Design review of the part built by this model. Coordinates are the model's own, in mm. Face numbers are marked on the shaded views. Give positions to 0.01 mm unless a question says otherwise; leave off trailing zeros.
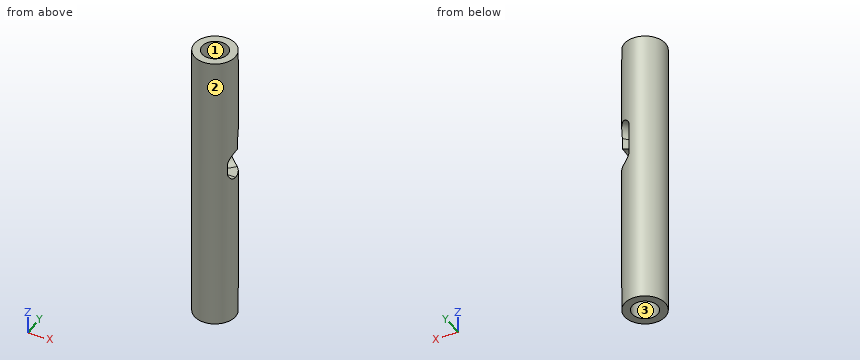
from build123d import *

# Parameters (mm, degrees)
SKETCH1_R           = 6.35
SKETCH1_R_2         = 3.2639
BOSS_EXTRUDE1_DEPTH = 88.9
CUT_EXTRUDE2_DEPTH  = 90.352420225
CUT_EXTRUDE3_DEPTH  = 90.352420338
SKETCH75_W          = 6.35
SKETCH75_H          = 6.35
CUT_REVOLVE1_ANGLE  = 45


# Read off the part's stored shape, not the designer's step: 3/8-16 Tapped Hole3
with BuildPart() as part:
    # Sketch1 → Boss-Extrude1 (new body)
    with BuildSketch(Plane.XY):
        Circle(SKETCH1_R)
        Circle(SKETCH1_R_2, mode=Mode.SUBTRACT)
    extrude(amount=BOSS_EXTRUDE1_DEPTH)

    # 3/8-16 Tapped Hole3 outline → 3/8-16 Tapped Hole3 (revolve, cut)
    with BuildSketch(Plane.XZ):
        Polygon((3.2639, 88.9), (3.2639, 69.426483393), (3.96875, 69.85), (3.96875, 88.9), align=None)
        Polygon((3.96875, 19.05), (3.2639, 19.473516607), (3.2639, 0), (3.96875, 0), align=None)
    revolve(axis=Axis((0, 0, 0), (0, 0, 1)), mode=Mode.SUBTRACT)

    # Sketch13 → Cut-Extrude2 (cut, through all)
    with BuildSketch(Plane(origin=(0, 0, 0), x_dir=(0, 0, -1), z_dir=(1, 0, 0))):
        with BuildLine():
            Line((-50.8, -3.175), (-53.34, -3.175))
            ThreePointArc((-53.34, -3.175), (-56.515, 0), (-53.34, 3.175))
            Line((-53.34, 3.175), (-50.8, 3.175))
            ThreePointArc((-50.8, 3.175), (-47.625, 0), (-50.8, -3.175))
        make_face()
    extrude(amount=CUT_EXTRUDE2_DEPTH, mode=Mode.SUBTRACT)

    # Sketch52 → Cut-Extrude3 (cut, through all)
    with BuildSketch(Plane(origin=(0, 0, 0), x_dir=(0.7071067811865491, -0.7071067811865461, 0), z_dir=(0.7071067811865461, 0.7071067811865491, 0))):
        with BuildLine():
            Line((3.175, -50.8), (3.175, -59.69))
            ThreePointArc((3.175, -59.69), (0, -62.865), (-3.175, -59.69))
            Line((-3.175, -59.69), (-3.175, -50.8))
            ThreePointArc((-3.175, -50.8), (0, -47.625), (3.175, -50.8))
        make_face()
    extrude(amount=CUT_EXTRUDE3_DEPTH, mode=Mode.SUBTRACT)

    # Sketch75 → Cut-Revolve1 (revolve, cut)
    with BuildSketch(Plane(origin=(0, 0, 0), x_dir=(1, 0, 0), z_dir=(0, 1, 0))):
        with Locations((3.175, -50.8)):
            Rectangle(SKETCH75_W, SKETCH75_H)
    revolve(axis=Axis((0, 0, 0), (0, 0, 1)), revolution_arc=CUT_REVOLVE1_ANGLE, mode=Mode.SUBTRACT)


solid = part.part
Q1. Wall thickness on line 1 (Y direction, x = 0, z = 6.75); line 2 (Y direction, x = 0, z = 41); line 3 (X direction, y = 0.25, z = 19): over which ranges is each line inside the solid? List them lowest first.
Results:
line 1: y = -6.35 to -3.97, 3.97 to 6.35
line 2: y = -6.35 to -3.26, 3.26 to 6.35
line 3: x = -6.35 to -3.96, 3.96 to 6.35
Q2. Insertion check: pin 1 (4 mm diameter, centred on x = 3.5, z = 62.5, fed in from +Y); pin 2 (2 mm diameter, centred on x = -4.5, z = 75, fed in from -Y); pin 3 (6 mm diameter, centred on x = 3.5, z = 54, fed in from -Y). Each pin has a flat end and moves straight along its axis. Give the tip position at first contact, or say it passes through.
Results:
pin 1: stops at y = 6.17
pin 2: stops at y = -5.3
pin 3: stops at y = -6.33
Q3. Draft analysis for pull direction Y (two halves, no side actions). For the marked faces 1, 2 and 3, state which applies: pulls with the +Y half, pulls with the -Y half, needs draft (parallel to the pull), parting line crosses it, or undercut.
Results:
face 1: undercut
face 2: parting line crosses it
face 3: undercut
